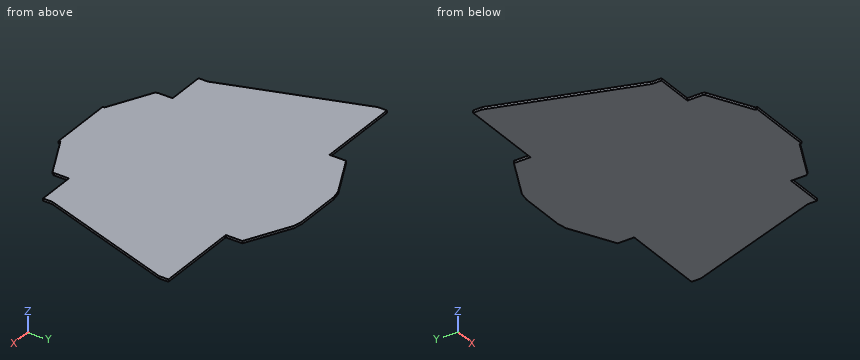
from build123d import *

# Parameters (mm, degrees)
BOSS_EXTRUDE1_DEPTH = 12.7


with BuildPart() as part:
    # Sketch1 → Boss-Extrude1 (new body)
    with BuildSketch(Plane.XY):
        Polygon((-207.569853327, -422.408510368), (-37.10675463, -422.408510368), (-37.10675463, -505.433281316), (-30.086367293, -516.792506642), (202.852470696, -633.261925636), (202.852470696, -642.963862322), (380.652470696, -642.963862322), (380.652470696, 661.746841587), (253.652470696, 661.746841587), (202.852470696, 652.044904901), (-37.10675463, 532.065292238), (-37.10675463, 441.191489632), (-461.569853327, 441.191489632), (-499.669853327, 441.191489632), (-499.669853327, 393.865899836), (-499.018131212, 388.436323288), (-245.669853327, -371.608510368), (-245.669853327, -422.408510368), align=None)
    extrude(amount=BOSS_EXTRUDE1_DEPTH)

    # Mirror1: part across plane


with BuildPart() as part_1:
    add(part.part)
    add(part.part.mirror(Plane(origin=(380.652470696, 661.746841587, 12.7), x_dir=(0, 0, 1), z_dir=(-1, 0, 0))))


solid = part_1.part
Geometry check sheet. Reference: the model listing, model coordinates, mm. Coordinates: 2 decimals unless noted, no trailing zeros. Loops run counter-clockwise (first coordinate to the right, second up) from the corner with the lowest first, then second, coordinate; pieces in that order, holes last. Notation, with made-up numbers: (-5.5, 77.5) - (32.5, 77.5) arc R17 ccw to (32.5, 108.5) - close; hole circle Ø11 at (29.25, 0.25). An arc over 180 degrees is marked (long way). Use one line per item in the form item = value. Start each with the question number.
Item 1: Section check A-A, the plane z = 3.75. Enter the section's corners in (x, y).
Item 2: Section check B-B, the plane x = -202. Enter the section's corners in (y, z).
Item 3: Thickness scan on probe 1 along X at (y, z) = (-458.5, 1); probe 2 along Y at (x, z) = (-41, 11.25); probe 3 along X at (y, z) = (-418.5, 7.75). Record the ranges inside material, lowest first.
Item 4: Gauge pin test, flat ends, axial feed: pin 1 (5 mm diameter, centred on x = -96, z = 8, fed in from +Y); pin 2 (6.5 mm diameter, centred on y = -456, z = 8, fed in from -X); pin 3 (6.5 mm diameter, centred on y = -400, z = 4.5, fed in from -X). Record the tip position at first contact, or that the pin passes through.
Item 5: Section check C-C, the plane y = 16.5. Enter the section's corners in (x, z).
Computed:
q1.outline = (-499.67, 393.87) - (-499.02, 388.44) - (-245.67, -371.61) - (-245.67, -422.41) - (-37.11, -422.41) - (-37.11, -505.43) - (-30.09, -516.79) - (202.85, -633.26) - (202.85, -642.96) - (558.45, -642.96) - (558.45, -633.26) - (791.39, -516.79) - (798.41, -505.43) - (798.41, -422.41) - (1006.97, -422.41) - (1006.97, -371.61) - (1260.32, 388.44) - (1260.97, 393.87) - (1260.97, 441.19) - (798.41, 441.19) - (798.41, 532.07) - (558.45, 652.04) - (507.65, 661.75) - (253.65, 661.75) - (202.85, 652.04) - (-37.11, 532.07) - (-37.11, 441.19) - (-499.67, 441.19) - close
q2.outline = (-422.41, 0) - (441.19, 0) - (441.19, 12.7) - (-422.41, 12.7) - close
q3.probe_1 = -37.11 to 798.41
q3.probe_2 = -422.41 to 441.19
q3.probe_3 = -245.67 to 1006.97
q4.pin_1 = 441.19
q4.pin_2 = -37.11
q4.pin_3 = -245.67
q5.outline = (-375.04, 0) - (1136.34, 0) - (1136.34, 12.7) - (-375.04, 12.7) - close
